Model file for the job. Use its own axes, mm. Face numbers are marked on the shaded views. A direction names the side the tool comes from. Coordinates: 2 decimals unless noted, no trailing zeros. Write each loop counter-clockwise with the first axis right and the second up, starting at its lowest first coordinate (ties: lowest second). Pieces come first, ordered by that corner, then holes. Notation, with made-up numbers: M 62,-27 L 97,-27 A12 cw 97,-11 Z; hole C 35.5,2 d10. An arc over 180 degrees is marked long. One line per question, with ' | ' between items. Start each with the question number.
(1) Wall check: probe 1 along Y at (x, z) = (-5.75, 0) (3 decimals); probe 2 along X at (y, z) = (-4.75, 2); probe 3 along X at (y, z) = (5.5, 1.75). Give the ranges that are in metal, low to high.
(2) Tool access for the marked faces 4 and 5: list every direction of +Z, -Z, +X, -X, +Y, -Y with a clear straight run to the whole face (end or side of a thin tool).
(3) Flat gauge pins, fed straight in: pin 1 Ø7.5 at (y, z) = (3, 1) entering from +X; pin 2 Ø1 at (x, y) = (-3, -2) entering from +Z; pin 3 Ø4 at (y, z) = (3, 2) entering from -X; pin 4 Ø1.5 at (y, z) = (4, 6) entering from +X. Where does each tip first touch, or does it go through?
(4) Cut at D-D (x = -0.25). Write the cut outline in (y, z), plus the area to 3 significant figures.
(5) Cut at A-A (x = -6.5). Write the cut outline in (y, z) (3 decimals).
(6) Cut at B-B (z = 0). Write the cut outline in (x, y) (3 decimals), plus the area to 3 significant figures.
(7) Two-plate mould, pull along Y, no slides. Class the marked faces 1, 2 and 3: +Y half, -Y half, draft (parallel to the pull), parting line (faces both ways), or undercut.
from build123d import *

# Parameters (mm, degrees)
SKETCH1_R           = 8.255
BOSS_EXTRUDE1_DEPTH = 12.7
SKETCH2_R           = 5.715
CUT_EXTRUDE1_DEPTH  = 10.16
CHAMFER1_SIZE       = 0.762


with BuildPart() as part:
    # Sketch1 → Boss-Extrude1 (new body)
    with BuildSketch(Plane(origin=(0, 0, 0), x_dir=(0, 0, -1), z_dir=(1, 0, 0))):
        Circle(SKETCH1_R)
    extrude(amount=-BOSS_EXTRUDE1_DEPTH)

    # Sketch2 → Cut-Extrude1 (cut)
    with BuildSketch(Plane.ZY.offset(12.7)):
        Circle(SKETCH2_R)
    extrude(amount=-CUT_EXTRUDE1_DEPTH, mode=Mode.SUBTRACT)

    # Chamfer1
    chamfer1_edges = [part.edges().sort_by_distance(p)[0] for p in [
        (0, 0, 8.255),
        (-12.7, 0, 8.255),
    ]]
    chamfer(chamfer1_edges, length=CHAMFER1_SIZE)

    # Sketch3 → Revolve1 (revolve)
    with BuildSketch(Plane(origin=(0, 0, 0), x_dir=(1, 0, 0), z_dir=(0, 1, 0))):
        Polygon((0, 0), (1.016, 0), (1.016, 2.54), (0, 3.556), align=None)
    revolve(axis=Axis((-11.938, 0, 0), (1, 0, 0)))


solid = part.part
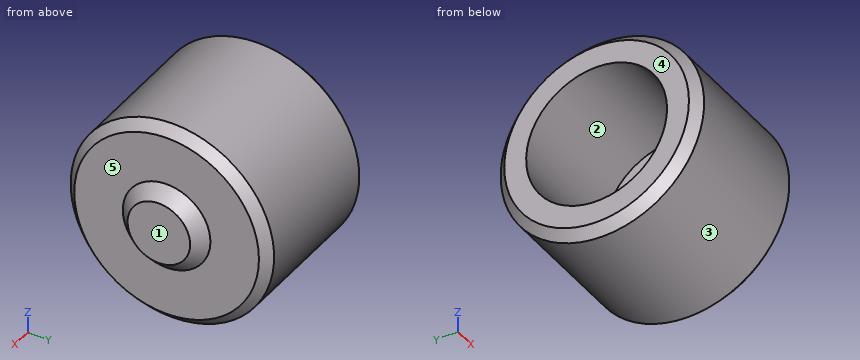
Filled in:
1) probe 1: -8.255 to -5.715, 5.715 to 8.255 | probe 2: -2.54 to 0 | probe 3: -12.7 to 0
2) face 4: +Z, -Z, -X, +Y, -Y | face 5: +X
3) pin 1: x = 1.02 | pin 2: z = 8.12 | pin 3: x = -2.54 | pin 4: x = 0
4) outline: C 0,0 d15.49 | area: 188 mm²
5) outline: C 0,0 d16.51; hole C 0,0 d11.43
6) outline: M -12.7,-7.493 L -11.938,-8.255 L -0.762,-8.255 L 0,-7.493 L 0,-3.556 L 1.016,-2.54 L 1.016,2.54 L 0,3.556 L 0,7.493 L -0.762,8.255 L -11.938,8.255 L -12.7,7.493 L -12.7,5.715 L -2.54,5.715 L -2.54,-5.715 L -12.7,-5.715 Z | area: 98.6 mm²
7) face 1: draft | face 2: undercut | face 3: parting line
